Here's the drawing with two shaded views (mm, measured from the low corner). I have some questions. A direction names the side the tool comes from. Coordinates: 2 decimals unless noted, no trailing zeros. Order: outer loops, then holes, each group sorted by start corner. A loop starts at its lowest first (then second) coordinate and runs counter-clockwise, first axis right, second up. Notation, with made-up numbers: (17, 29.5) - (76, 29.5) arc R28 cw to (76, 66.5) - close; hole circle Ø7 at (65.25, -19). An arc over 180 degrees is marked (long way). Answer as a JSON object with one key per item and string values. Group by question number.
(1) Imagine slicing it at C-C, the plane x = 8. Write out the boundary of the cut face in (y, z).
(2) Imagine slicing it at A-A, the plane z = 10. Write out the boundary of the cut face in (x, y).
(3) We'd pull the mould along Y, two halves only. Please class the marked faces 3, 4 and 5: pulls with the +Y half, pulls with the -Y half, needs draft (parallel to the pull), parting line crosses it, or undercut.
(4) Imagine slicing it at B-B, the plane y = 12. Write out the boundary of the cut face in (x, z), and give its area (3 significant figures).
(5) Which directions (+Z, -Z, +X, -X, +Y, -Y) give clear straight access to the entire face, cutting with the end or side of a thin tool? Please do the marked faces 1 and 2.
(6) Imagine slicing it at D-D, the plane x = 15.25. Write out the boundary of the cut face in (y, z), and give its area (3 significant figures).
(7) Will these pins go through, and if not, where does the flat tip stop? P1, Ø2, axis at x = 4, z = 12.5, coming from the +Y side; P2, Ø6, axis at y = 11, z = 16, coming from the -X side; P3, Ø1, axis at y = 7, z = 5.5, coming from the -X side.
(8) Please list where these lines run through material, in increasing order: probe 1 along Z at (x, y) = (8, 2.65); probe 2 along Z at (x, y) = (9.25, 7.25); probe 3 along Y at (x, z) = (18.35, 10).
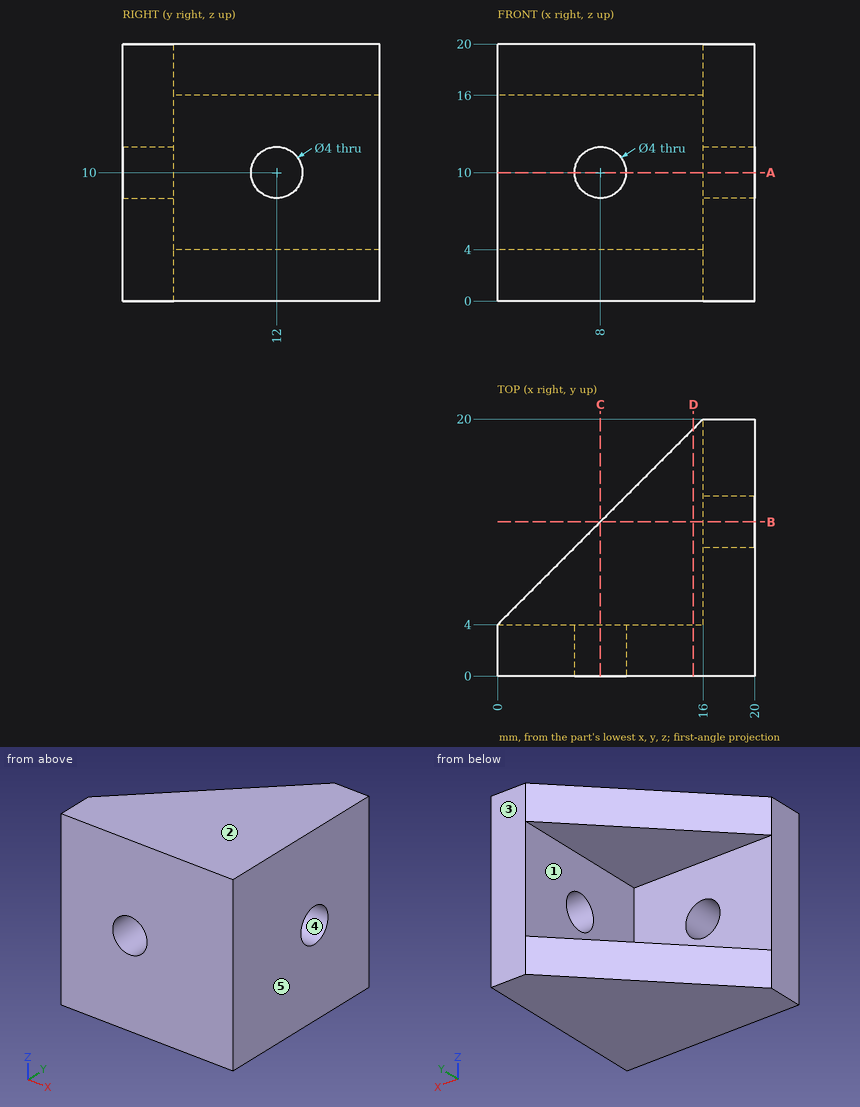
Result set:
{
 "1": {"outline": "(0, 0) - (12, 0) - (12, 4) - (4, 4) - (4, 8) - (0, 8) - close; (0, 12) - (4, 12) - (4, 16) - (12, 16) - (12, 20) - (0, 20) - close"},
 "2": {"outline": "(0, 0) - (6, 0) - (6, 4) - (0, 4) - close; (10, 0) - (20, 0) - (20, 10) - (16, 10) - (16, 4) - (10, 4) - close; (16, 14) - (20, 14) - (20, 20) - (16, 20) - close"},
 "3": {"face 3": "pulls with the +Y half", "face 4": "undercut", "face 5": "needs draft"},
 "4": {"outline": "(8, 0) - (20, 0) - (20, 8) - (16, 8) - (16, 4) - (8, 4) - close; (8, 16) - (16, 16) - (16, 12) - (20, 12) - (20, 20) - (8, 20) - close", "area": "128 mm^2"},
 "5": {"face 1": "-X, +Y", "face 2": "+Z, +X, -X, +Y, -Y"},
 "6": {"outline": "(0, 0) - (19.25, 0) - (19.25, 4) - (4, 4) - (4, 16) - (19.25, 16) - (19.25, 20) - (0, 20) - close", "area": "202 mm^2"},
 "7": {"P1": "stops at y = 4", "P2": "stops at x = 4", "P3": "stops at x = 16"},
 "8": {"probe 1": "z = 0 to 8, 12 to 20", "probe 2": "z = 0 to 4, 16 to 20", "probe 3": "y = 0 to 10, 14 to 20"}
}
